```python
from build123d import *

# Parameters (mm, degrees)
F0_W     = 11.0358623788
F0_H     = 14.8984193802
F1_DEPTH = 25.4
F2_DEPTH = 25.4
F3_R     = 2.5571153932
F3_R_2   = 2.5440351013
F3_W     = 14.7031287464
F3_H     = 3.2673614761
F4_DEPTH = 25.4


# Not quite as in the source:
# - the program builds the solid bodies; features that only make, move or delete a surface that nothing else refers to are left out


with BuildPart() as f1:
    # F0 (on Right) → F1 (new body)
    with BuildSketch(Plane.YZ):
        with BuildLine():
            ThreePointArc((-24.4896995825, -21.3687317689), (-22.0066937129, -69.3902825337), (19.2165729762, -44.633931036))
            ThreePointArc((19.2165729762, -44.633931036), (14.5664371428, -29.167684068), (2.1580914014, -18.8302997515))
            ThreePointArc((2.1580914014, -18.8302997515), (-10.7088530026, -24.8964679727), (-24.4896995825, -21.3687317689))
        make_face()
        with BuildLine():
            ThreePointArc((-24.4896995825, -21.3687317689), (-10.7088530026, -24.8964679727), (2.1580914014, -18.8302997515))
            ThreePointArc((2.1580914014, -18.8302997515), (-11.4882033251, -16.7150534797), (-24.4896995825, -21.3687317689))
        make_face()
        with BuildLine():
            ThreePointArc((-24.4896995825, -21.3687317689), (-11.4882033251, -16.7150534797), (2.1580914014, -18.8302997515))
            ThreePointArc((2.1580914014, -18.8302997515), (6.7017838768, -12.0221001394), (8.2971597307, -3.993931036))
            ThreePointArc((8.2971597307, -3.993931036), (4.6343580327, 7.8551511373), (-5.0761488644, 15.5702610153))
            ThreePointArc((-5.0761488644, 15.5702610153), (-13.5382573111, 12.2302712352), (-22.2995232661, 14.6803793882))
            ThreePointArc((-22.2995232661, 14.6803793882), (-33.6585141964, -2.7205891991), (-24.4896995825, -21.3687317689))
        make_face()
        with BuildLine():
            ThreePointArc((-26.3456820786, 34.106068964), (-28.2496986989, 23.5752529976), (-22.2995232661, 14.6803793882))
            ThreePointArc((-22.2995232661, 14.6803793882), (-13.7834170108, 16.9752588467), (-5.0761488644, 15.5702610153))
            ThreePointArc((-5.0761488644, 15.5702610153), (-1.3310983759, 20.4668881546), (0, 26.486068964))
            ThreePointArc((0, 26.486068964), (-0.5620509112, 30.4522310833), (-2.2039436985, 34.106068964))
            Line((-2.2039436985, 34.106068964), (-26.3456820786, 34.106068964))
        make_face()
        with BuildLine():
            ThreePointArc((-5.0761488644, 15.5702610153), (-13.7834170108, 16.9752588467), (-22.2995232661, 14.6803793882))
            ThreePointArc((-22.2995232661, 14.6803793882), (-13.5382573111, 12.2302712352), (-5.0761488644, 15.5702610153))
        make_face()
        with BuildLine():
            Line((-28.4173451364, 34.106068964), (-26.3456820786, 34.106068964))
            ThreePointArc((-26.3456820786, 34.106068964), (-14.2748128886, 40.7608818526), (-2.2039436985, 34.106068964))
            Line((-2.2039436985, 34.106068964), (0, 34.106068964))
            Line((0, 34.106068964), (0, 41.5552749288))
            Line((0, 41.5552749288), (-9.9322767928, 41.5552749288))
            Line((-9.9322767928, 41.5552749288), (-20.9681391716, 41.5552749288))
            Line((-20.9681391716, 41.5552749288), (-28.4173451364, 41.5552749288))
            Line((-28.4173451364, 41.5552749288), (-28.4173451364, 34.106068964))
        make_face()
        with BuildLine():
            ThreePointArc((-2.2039436985, 34.106068964), (-14.2748128886, 40.7608818526), (-26.3456820786, 34.106068964))
            Line((-26.3456820786, 34.106068964), (-2.2039436985, 34.106068964))
        make_face()
        with Locations((-15.4502079822, 49.0044846189)):
            Rectangle(F0_W, F0_H)
    extrude(amount=F1_DEPTH)

    # F0 (on Right) → F2 (join)
    with BuildSketch(Plane.YZ):
        with BuildLine():
            ThreePointArc((-24.4896995825, -21.3687317689), (-22.0066937129, -69.3902825337), (19.2165729762, -44.633931036))
            ThreePointArc((19.2165729762, -44.633931036), (14.5664371428, -29.167684068), (2.1580914014, -18.8302997515))
            ThreePointArc((2.1580914014, -18.8302997515), (-10.7088530026, -24.8964679727), (-24.4896995825, -21.3687317689))
        make_face()
        with BuildLine():
            ThreePointArc((-24.4896995825, -21.3687317689), (-10.7088530026, -24.8964679727), (2.1580914014, -18.8302997515))
            ThreePointArc((2.1580914014, -18.8302997515), (-11.4882033251, -16.7150534797), (-24.4896995825, -21.3687317689))
        make_face()
        with BuildLine():
            ThreePointArc((-24.4896995825, -21.3687317689), (-11.4882033251, -16.7150534797), (2.1580914014, -18.8302997515))
            ThreePointArc((2.1580914014, -18.8302997515), (6.7017838768, -12.0221001394), (8.2971597307, -3.993931036))
            ThreePointArc((8.2971597307, -3.993931036), (4.6343580327, 7.8551511373), (-5.0761488644, 15.5702610153))
            ThreePointArc((-5.0761488644, 15.5702610153), (-13.5382573111, 12.2302712352), (-22.2995232661, 14.6803793882))
            ThreePointArc((-22.2995232661, 14.6803793882), (-33.6585141964, -2.7205891991), (-24.4896995825, -21.3687317689))
        make_face()
        with BuildLine():
            ThreePointArc((-26.3456820786, 34.106068964), (-28.2496986989, 23.5752529976), (-22.2995232661, 14.6803793882))
            ThreePointArc((-22.2995232661, 14.6803793882), (-13.7834170108, 16.9752588467), (-5.0761488644, 15.5702610153))
            ThreePointArc((-5.0761488644, 15.5702610153), (-1.3310983759, 20.4668881546), (0, 26.486068964))
            ThreePointArc((0, 26.486068964), (-0.5620509112, 30.4522310833), (-2.2039436985, 34.106068964))
            Line((-2.2039436985, 34.106068964), (-26.3456820786, 34.106068964))
        make_face()
        with BuildLine():
            ThreePointArc((-5.0761488644, 15.5702610153), (-13.7834170108, 16.9752588467), (-22.2995232661, 14.6803793882))
            ThreePointArc((-22.2995232661, 14.6803793882), (-13.5382573111, 12.2302712352), (-5.0761488644, 15.5702610153))
        make_face()
        with BuildLine():
            Line((-28.4173451364, 34.106068964), (-26.3456820786, 34.106068964))
            ThreePointArc((-26.3456820786, 34.106068964), (-14.2748128886, 40.7608818526), (-2.2039436985, 34.106068964))
            Line((-2.2039436985, 34.106068964), (0, 34.106068964))
            Line((0, 34.106068964), (0, 41.5552749288))
            Line((0, 41.5552749288), (-9.9322767928, 41.5552749288))
            Line((-9.9322767928, 41.5552749288), (-20.9681391716, 41.5552749288))
            Line((-20.9681391716, 41.5552749288), (-28.4173451364, 41.5552749288))
            Line((-28.4173451364, 41.5552749288), (-28.4173451364, 34.106068964))
        make_face()
        with BuildLine():
            ThreePointArc((-2.2039436985, 34.106068964), (-14.2748128886, 40.7608818526), (-26.3456820786, 34.106068964))
            Line((-26.3456820786, 34.106068964), (-2.2039436985, 34.106068964))
        make_face()
        with Locations((-15.4502079822, 49.0044846189)):
            Rectangle(F0_W, F0_H)
    extrude(amount=F2_DEPTH)

    # F3 (on Right) → F4 (cut)
    with BuildSketch(Plane.YZ):
        with Locations((-20.32, 31.496)):
            Circle(F3_R)
        with Locations((-8.89, 31.4950787105)):
            Circle(F3_R_2)
        with Locations((-13.7015643732, 19.5692073871)):
            Rectangle(F3_W, F3_H)
    extrude(amount=F4_DEPTH, mode=Mode.SUBTRACT)


solid = f1.part
```
Source: CAD feature listing. Evaluate the final solid. Frame: model axes, mm. A direction names the side the tool comes from. Round coordinates to 2 decimals unless told otherwise and drop trailing zeros. Loops run counter-clockwise (first coordinate to the right, second up) from the corner with the lowest first, then second, coordinate; pieces in that order, holes last. Notation, with made-up numbers: M 64.25,-22 L 123.25,-22 A19 ccw 123.25,-12 Z; hole C -8.75,56.25 d7. An arc over 180 degrees is marked long. Use a Markdown table: item, result. Add a question column.
1. Contact query for flat-ended pins moving along their axis: pin 1 (0.6 mm diameter, centred on x = 18, y = -27.5, fed in from -Z); pin 2 (3 mm diameter, centred on x = 4.5, y = 1, fed in from -Z); pin 3 (1 mm diameter, centred on x = 5.5, y = -15.5, fed in from -Z). Output: stop coordinate, or through.
2. Cut plane A-A, the plane z = 20. Output: boundary loops of the cut face in (x, y).
3. Cut plane C-C, the plane z = -6.5. Output: boundary loops of the cut face in (x, y).
4. Pull-direction query (Z, two-part tool) for faces 4 (the flat face through (13, -25, 41.555)), 5 (the flat face through (13, -1, 34.106)), 6 (the flat face through (13, -20.968, 49)); classes: +Z half, -Z half, draft (parallel to the pull), parting line (faces both ways), or undercut.
5. Cut plane B-B, the plane x = 20. Output: boundary loops of the cut face in (y, z), and give its area (3 significant figures).
6. Set-up query: faces 1 (the flat face through (13, -6.35, 20)), 2 (the flat face through (13, 0, 38)), 3 (the flat face through (13, -28.417, 38)). Return all of +Z, -Z, +X, -X, +Y, -Y with unobstructed straight access to the full face (end or side cutting, diameter ignored); none if empty.
7. Ray query, line 1 along Z through (x, y) = (8.25, -8.89); line 2 along Z through (x, y) = (7.25, -20.32); line 3 along Y through (x, z) = (13, 30). Return the intervals inside material, ascending. Write a range as [from, to].
Solution:
| question | item | result |
|---|---|---|
| 1 | pin 1 | stops at z = -65.82 |
| 1 | pin 2 | stops at z = -71.41 |
| 1 | pin 3 | stops at z = -71.99 |
| 2 | outline | M 0,-26.99 L 25.4,-26.99 L 25.4,-21.05 L 0,-21.05 Z; M 0,-6.35 L 25.4,-6.35 L 25.4,-1.56 L 0,-1.56 Z |
| 3 | outline | M 0,-33.55 L 25.4,-33.55 L 25.4,8.15 L 0,8.15 Z |
| 4 | face 4 | +Z half |
| 4 | face 5 | undercut |
| 4 | face 6 | draft |
| 5 | outline | M -28.42,34.11 L -26.35,34.11 A14.27 ccw -22.3,14.68 A21 ccw -24.49,-21.37 A28.05 ccw long 2.16,-18.83 A21 ccw -5.08,15.57 A14.27 ccw -2.2,34.11 L 0,34.11 L 0,41.56 L -9.93,41.56 L -9.93,56.45 L -20.97,56.45 L -20.97,41.56 L -28.42,41.56 Z; hole C -20.32,31.5 d5.11; hole M -21.05,17.94 L -6.35,17.94 L -6.35,21.2 L -21.05,21.2 Z; hole C -8.89,31.5 d5.09 |
| 5 | area | 4,460 mm2 |
| 6 | face 1 | +X, -X |
| 6 | face 2 | +Z, +X, -X, +Y |
| 6 | face 3 | +Z, +X, -X, -Y |
| 7 | line 1 | z = [-72.68, 17.94], [21.2, 28.95], [34.04, 41.56] |
| 7 | line 2 | z = [-70.22, 17.94], [21.2, 28.94], [34.05, 56.45] |
| 7 | line 3 | y = [-28.11, -22.39], [-18.25, -10.95], [-6.83, -0.44] |
